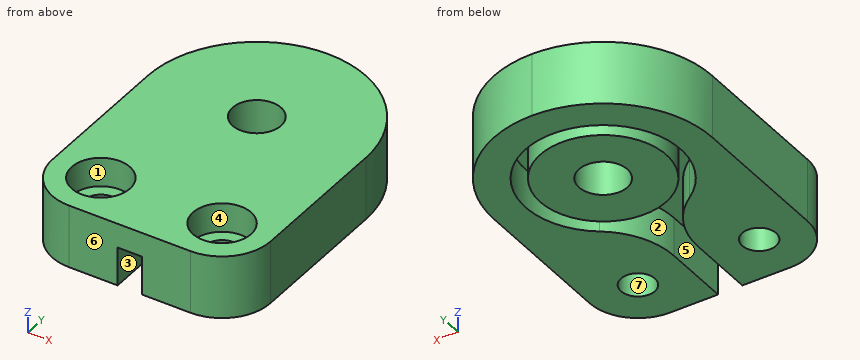
Autodesk Inventor part; units mm, degrees
ref_plane "YZ Plane" through (0, 0, 0) normal (1, 0, 0) x (0, 1, 0)
ref_plane "XZ Plane" through (0, 0, 0) normal (0, 1, 0) x (-1, 0, 0)
ref_plane "XY Plane" through (0, 0, 0) normal (0, 0, 1) x (1, 0, 0)
sketch "Sketch1" plane through (0, 0, 0) normal (0, 0, 1) x (1, 0, 0)
  line L0 (-1.25, 0) -> (1.25, 0)
  line L1 (-1.25, 0) -> (-1.25, 7)
  arc A0 (-1.25, 7) -> (-4.625, 13.5276) centre (-9.25, 7) ccw
  arc A1 (4.625, 13.5276) -> (-4.625, 13.5276) centre (0, 20.0552) ccw
  arc A2 (4.625, 13.5276) -> (1.25, 7) centre (9.25, 7) ccw
  line L2 (1.25, 7) -> (1.25, 0)
  circle A3 centre (0, 20.0552) radius 6.5
  line L3 (-1.25, 0) -> (-11.25, 0)
  line L4 (-11.25, 0) -> (-11.25, 31.3052)
  line L5 (-11.25, 31.3052) -> (11.25, 31.3052)
  line L6 (11.25, 31.3052) -> (11.25, 0)
  line L7 (11.25, 0) -> (1.25, 0)
  point P0 (0, 0)
  point P1 (0, 0)
  dimension "d0" = 2.5
  dimension "d3" = 7
  dimension "d4" = 1.5
  dimension "d15" = 10
  dimension "d23" = 11.25
  dimension "d24" = 8
extrude "Extrusion1" add sketch "Sketch1" along normal blind 6.5 contours L3 L4 L5 L6 L7 L2 A2 A1 A0 L1 | A3
fillet "Fillet1" radius 11.25 2 edges at (11.25, 31.3052, 3.25) (-11.25, 31.3052, 3.25)
sketch "Sketch2" plane through (0, 0, 6.5) normal (0, 0, 1) x (1, 0, 0)
  line L0 (-1.25, 0) -> (-1.25, 7)
  arc A0 (-1.25, 7) -> (-4.625, 13.5276) centre (-9.25, 7) ccw
  arc A1 (4.625, 13.5276) -> (-4.625, 13.5276) centre (0, 20.0552) ccw
  arc A2 (4.625, 13.5276) -> (1.25, 7) centre (9.25, 7) ccw
  line L1 (1.25, 7) -> (1.25, 0)
  line L2 (11.25, 0) -> (11.25, 20.0552)
  line L3 (-1.25, 0) -> (1.25, 0)
  point P0 (0, 0)
extrude "Extrusion2" add sketch "Sketch2" against normal blind 2.5
sketch "Sketch3" plane through (0, 0, 0) normal (0, 0, -1) x (-1, 0, 0)
  line L0 (-1.25, 0) -> (-11.25, 0)
  line L1 (11.25, 0) -> (1.25, 0)
  circle A0 centre (-6.25, 5) radius 1.75
  circle A1 centre (6.25, 5) radius 1.75
  point P0 (0, 0)
  point P1 (-1.25, 22.4355)
  point P2 (-6.25, 0)
  point P3 (6.25, 0)
  dimension "d13" = 5
  dimension "d14" = 3.5
extrude "Extrusion3" cut sketch "Sketch3" against normal through all
sketch "Sketch4" plane through (0, 0, 6.5) normal (0, 0, 1) x (1, 0, 0)
  circle A0 centre (6.25, 5) radius 1.75
  circle A1 centre (-6.25, 5) radius 1.75
  circle A2 centre (-6.25, 5) radius 3
  circle A3 centre (6.25, 5) radius 3
  point P0 (0, 0)
  dimension "d19" = 6
extrude "Extrusion4" cut sketch "Sketch4" against normal blind 3
fillet "Fillet2" radius 5 2 edges at (-11.25, 0, 3.25) (11.25, 0, 3.25)
sketch "Sketch5" plane through (0, 0, 6.5) normal (0, 0, 1) x (1, 0, 0)
  arc A0 (11.25, 20.0552) -> (-11.25, 20.0552) centre (0, 20.0552) ccw
  circle A1 centre (0, 20.0552) radius 2.5
  point P0 (0, 0)
  dimension "d26" = 5
extrude "Extrusion5" cut sketch "Sketch5" against normal through all
equation "\"d9\" = d16"
properties part number "belt tensioner"
CAD build for the part. Positions are in the model's coordinates, mm. Face numbers are marked on the shaded views. A direction names the side the tool comes from. Coordinates: 2 decimals unless noted, no trailing zeros. Order: outer loops, then holes, each group sorted by start corner. A loop starts at its lowest first (then second) coordinate and runs counter-clockwise, first axis right, second up. Notation, with made-up numbers: (75, 53) - (116, 53) arc R21 cw to (116, 83) - close; hole circle Ø2 at (40.25, 32). An arc over 180 degrees is marked (long way). Answer in a Markdown table with one row per item.
1. Drill centre lines: L1, parallel to X at y = 5, z = 0.75; L2, parallel to Y at x = -5.75, z = 0.5; L3, parallel to Y at x = 0, z = 2.5. Where is each one in solid material? Low to high. Write a range as from..to.
Answer:
| item | result |
|---|---|
| L1 | -11.25..-8, -4.5..-1.25, 1.25..4.5, 8..11.25 |
| L2 | 0..3.32, 6.68..14.49, 17.02..23.09, 25.62..29.72 |
| L3 | 13.56..17.56, 22.56..26.56, 28.06..31.31 |
2. 3-axis set-ups, long thin cutter, end or side, ignore diameter. For the marked faces 1, 2 and 3: which of +Z, -Z, +X, -X, +Y, -Y reach the whole face in a straight line?
Answer:
| item | result |
|---|---|
| face 1 | +Z |
| face 2 | -Z |
| face 3 | -Z, -Y |
3. Flat gauge pins, fed straight in: P1, Ø2, axis at y = 22, z = 5.5, coming from the +X side; P2, Ø2, axis at y = 3.5, z = 3, coming from the -X side. Where does each tip first touch, or does it go through?
Answer:
| item | result |
|---|---|
| P1 | x = 11.21 |
| P2 | x = -11.22 |
4. Slice it at A-A, the plane z = 2.5. Give the number of separate pieces and of enclosed holes in the cut face, then the cut area to 3 significant figures.
Answer:
| item | result |
|---|---|
| separate pieces | 2 |
| enclosed holes | 3 |
| area | 494 mm² |
5. Pull direction Y, two halves, no side cores. Call the marked faces 4, 5, 6 and 7: +Y half, -Y half, draft (parallel to the pull), parting line (faces both ways), or undercut.
Answer:
| item | result |
|---|---|
| face 4 | undercut |
| face 5 | draft |
| face 6 | -Y half |
| face 7 | undercut |
6. Slice it at B-B, the plane y = 9.5. List the corners of the cut face in (x, z).
Answer:
| item | result |
|---|---|
| outline | (-11.25, 0) - (-1.65, 0) - (-1.65, 4) - (1.65, 4) - (1.65, 0) - (11.25, 0) - (11.25, 6.5) - (-11.25, 6.5) - close |
